Can you work these out from the model? Positions are in its coordinate system, mm. Face numbers are marked on the shaded views. A direction names the side the tool comes from. Round coordinates to 2 decimals unless told otherwise and drop trailing zeros. Order: outer loops, then holes, each group sorted by start corner. A loop starts at its lowest first (then second) coordinate and runs counter-clockwise, first axis right, second up. Notation, with made-up numbers: M -29,-20.5 L 2,-20.5 A23 cw 2,3.5 Z; hole C -23,30.5 d9. An arc over 180 degrees is marked long. Answer as CSV lines item,"result". Start each with the question number.
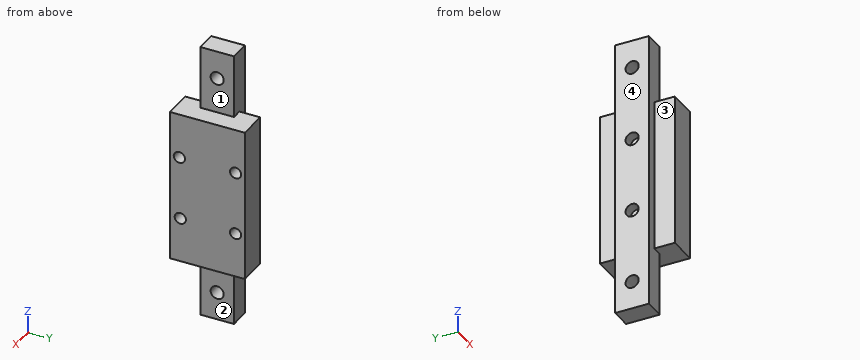
Autodesk Inventor part; units mm, degrees
ref_plane "YZ Plane" through (0, 0, 0) normal (1, 0, 0) x (0, 1, 0)
ref_plane "XZ Plane" through (0, 0, 0) normal (0, 1, 0) x (-1, 0, 0)
ref_plane "XY Plane" through (0, 0, 0) normal (0, 0, 1) x (1, 0, 0)
sketch "Skizze1" plane through (0, 0, 0) normal (1, 0, 0) x (0, 1, 0)
  line L0 (0, 0) -> (9, 0)
  line L1 (9, 0) -> (9, 75)
  line L2 (9, 75) -> (0, 75)
  line L3 (0, 75) -> (0, 0)
  dimension "d0" = 9
  dimension "d1" = 75
extrude "Extrusion1" add sketch "Skizze1" along normal blind 5.5
sketch "Skizze2" plane through (5.5, 0, 0) normal (1, 0, 0) x (0, 0, -1)
  line L0 (0, 0) -> (0, 9)
  line L1 (0, 9) -> (-75, 9)
  line L2 (-75, 9) -> (-75, 0)
  line L3 (-75, 0) -> (0, 0)
  circle A0 centre (-67.5, 4.5) radius 1.75
  circle A1 centre (-7.5, 4.5) radius 1.75
  circle A2 centre (-47.5, 4.5) radius 1.75
  circle A3 centre (-27.5, 4.5) radius 1.75
  dimension "d4" = 3.5
  dimension "d5" = 7.5
  dimension "d6" = 3.5
  dimension "d7" = 7.5
  dimension "d8" = 3.5
  dimension "d9" = 20
  dimension "d10" = 3.5
  dimension "d11" = 20
extrude "Extrusion2" cut sketch "Skizze2" against normal through all contours A0 | A1 | A2 | A3
sketch "Skizze3" plane through (5.5, 0, 0) normal (1, 0, 0) x (0, 0, -1)
  circle A0 centre (-47.5, 4.5) radius 1.75
  circle A1 centre (-67.5, 4.5) radius 1.75
  circle A2 centre (-7.5, 4.5) radius 1.75
  circle A3 centre (-27.5, 4.5) radius 1.75
  line L0 (0, 0) -> (0, 9)
  line L1 (0, 9) -> (-75, 9)
  line L2 (-75, 9) -> (-75, 0)
  line L3 (-75, 0) -> (0, 0)
  line L4 (-58, 14.5) -> (-17, 14.5)
  line L5 (-17, 14.5) -> (-17, -5.5)
  line L6 (-17, -5.5) -> (-58, -5.5)
  line L7 (-58, -5.5) -> (-58, 14.5)
  line L8 (-58, 14.5) -> (-17, -5.5) construction
  line L9 (-17, 14.5) -> (-58, -5.5) construction
  point P0 (-37.5, 4.5)
  dimension "d15" = 41
  dimension "d16" = 20
extrude "Extrusion3" add sketch "Skizze3" along normal blind 5 and the other way blind 2.75 contours A0 | A3 | L5 L6 L7 L3 | L3 L7 L1 L5 | L1 L7 L4 L5
sketch "Skizze4" plane through (10.5, 0, 0) normal (1, 0, 0) x (0, 0, -1)
  line L0 (-17, 14.5) -> (-58, 14.5)
  line L1 (-58, 14.5) -> (-58, -5.5)
  line L2 (-58, -5.5) -> (-17, -5.5)
  line L3 (-17, -5.5) -> (-17, 14.5)
  circle A0 centre (-46, -3) radius 1.5
  circle A1 centre (-46, 12) radius 1.5
  circle A2 centre (-29, -2.75) radius 1.5
  circle A3 centre (-29, 12) radius 1.5
  circle A4 centre (-29, -2.75) radius 1.5
  circle A5 centre (-29, 12) radius 1.5
  circle A6 centre (-46, 12) radius 1.5
  circle A7 centre (-46, -3) radius 1.5
  line L4 (-23, -4.9525) -> (-23, 23.5)
  line L5 (-23, 23.5) -> (-58, 23.5)
  line L6 (-58, 23.5) -> (-58, -4.9525)
  line L7 (-23, -4.9525) -> (-58, -4.9525)
  circle A8 centre (-46, 21.0354) radius 1.5
  circle A9 centre (-30.5, 21.0354) radius 1.5
  circle A10 centre (-46, 20.5472) radius 1.5
  circle A11 centre (-30.5, 20.5472) radius 1.5
  point P0 (0, 0)
  dimension "d21" = 3
  dimension "d22" = 3
  dimension "d23" = 3
  dimension "d24" = 3
  dimension "d27" = 3
  dimension "d28" = 3
extrude "Extrusion4" cut sketch "Skizze4" against normal blind 5 contours A0 | A1 | A2 | A3 | A8 A10 | A10 A8 | A9 A11 | A11 A9 picked at (-46.157, 22.1946) picked at (-45.8838, 21.1962) picked at (-30.657, 22.1946) picked at (-30.3838, 20.3864)
properties part number "90_Linearführung" material "Eisen, grau"
(1) If I drill on line 1 along Y through (x, z) = (6.7, 29); line 2 along Y through (x, z) = (1.8, 7.5); line 3 along X through (y, z) = (4.75, 58.5), over which ranges is the centre line in solid material (lowest first)?
(2) I want a section at B-B on x = 8.25. Write out the boundary of the cut face in (y, z).
(3) I want a section at C-C on y = 4.5. Write out the boundary of the cut face in (x, z).
(4) For the marked faces 1, 2, 3 and 4, which set-ups out of +Z, -Z, +X, -X, +Y, -Y let a thin tool reach every point of the face, with its end or its side?
(5) I want a section at A-A on z = 7.5. Write out the boundary of the cut face in (x, y).
(6) I want a section at D-D on x = 4. Write out the boundary of the cut face in (y, z), and give its area (3 significant figures).
(7) I'm going to push flat-ended pins straight in: P1, Ø0.9, axis at y = 11.5, z = 29, coming from the +X side; P2, Ø3, axis at x = 9.5, y = 5, coming from the -Z side; P3, Ø4, axis at y = 12, z = 29, coming from the -X side. Where does each tip first touch, or does it pass through?
From the geometry:
1,line 1,"-5.5 to -4.25, -1.25 to 10.5, 13.5 to 14.5"
1,line 2,"0 to 2.75, 6.25 to 9"
1,line 3,"0 to 5.5"
2,outline,"M -5.5,17 L 14.5,17 L 14.5,58 L -5.5,58 Z; hole C -3,46 d3; hole C -2.75,29 d3; hole C 12,29 d3; hole C 12,46 d3"
3,outline,"M 0,0 L 5.5,0 L 5.5,5.75 L 0,5.75 Z; M 0,9.25 L 5.5,9.25 L 5.5,17 L 10.5,17 L 10.5,58 L 5.5,58 L 5.5,65.75 L 0,65.75 L 0,49.25 L 2.75,49.25 L 2.75,45.75 L 0,45.75 L 0,29.25 L 2.75,29.25 L 2.75,25.75 L 0,25.75 Z; M 0,69.25 L 5.5,69.25 L 5.5,75 L 0,75 Z"
4,face 1,"+Z, +X, +Y, -Y"
4,face 2,"-Z, +X, +Y, -Y"
4,face 3,"+Z, -Z, -X, -Y"
4,face 4,"+Z, -Z, -X, +Y, -Y"
5,outline,"M 0,0 L 5.5,0 L 5.5,2.75 L 0,2.75 Z; M 0,6.25 L 5.5,6.25 L 5.5,9 L 0,9 Z"
6,outline,"M -5.5,17 L 0,17 L 0,0 L 9,0 L 9,17 L 14.5,17 L 14.5,58 L 9,58 L 9,75 L 0,75 L 0,58 L -5.5,58 Z; hole C 4.5,7.5 d3.5; hole C 4.5,67.5 d3.5"
6,area,"1,110 mm²"
7,P1,"x = 5.5"
7,P2,"z = 17"
7,P3,"x = 2.75"
